from build123d import *

# Parameters (mm, degrees)
F0_W     = 10
F0_H     = 10
F0_W_2   = 8
F0_H_2   = 8
F1_DEPTH = 250
F2_R     = 1.5
F4_DEPTH = 25
F3_R     = 1.5
F3_R_2   = 2.5
F5_DEPTH = 25


with BuildPart() as f1:
    # F0 (on Front) → F1 (new body)
    with BuildSketch(Plane.XZ):
        Rectangle(F0_W, F0_H)
        Rectangle(F0_W_2, F0_H_2, mode=Mode.SUBTRACT)
    extrude(amount=F1_DEPTH)

    # F2 (on face) → F4 (cut)
    with BuildSketch(Plane.YZ.offset(5)):
        with Locations((-140.5, -1)):
            Circle(F2_R)
        with Locations((-109.5, -1)):
            Circle(F2_R)
        with Locations((-235, 0)):
            Circle(F2_R)
        with Locations((-15, 0)):
            Circle(F2_R)
    extrude(amount=-F4_DEPTH, mode=Mode.SUBTRACT)

    # F3 (on face) → F5 (cut)
    with BuildSketch(Plane.XY.offset(5)):
        with Locations((0, -245)):
            Circle(F3_R)
        with Locations((0, -5)):
            Circle(F3_R)
        with Locations((0, -215)):
            Circle(F3_R_2)
        with Locations((0, -189)):
            Circle(F3_R_2)
        with Locations((0, -61)):
            Circle(F3_R_2)
        with Locations((0, -35)):
            Circle(F3_R_2)
    extrude(amount=-F5_DEPTH, mode=Mode.SUBTRACT)


solid = f1.part
Input: part model. Units: mm. Frame: model coordinates. A direction names the side the tool comes from. Coordinates: 2 decimals unless noted, no trailing zeros. Loops run counter-clockwise (first coordinate to the right, second up) from the corner with the lowest first, then second, coordinate; pieces in that order, holes last. Notation, with made-up numbers: (-5, 12) - (37, 12) arc R5 ccw to (37, 19) - close; hole circle Ø8 at (72, 83). An arc over 180 degrees is marked (long way). Answer in a Markdown table with one row per item. Add a question column.
Item 1: Section query B-B on y = -45.5. Return the cut outline in (x, z).
Item 2: Section query A-A on y = -189. Return the cut outline in (x, z).
Item 3: Contact query for a flat-ended pin moving along its axis: P1, Ø3, axis at x = -0.5, z = -1.5, coming from the -Y side. Output: stop coordinate, or through.
Item 4: Mould query, pull axis Y, two halves, no side actions, for faces 1 (the cylindrical face through (-0.33, -186.52, 4.51)), 2 (the cylindrical face through (1.34, -32.89, 4.51)), 3 (the flat face through (0, -123, 5)), 4 (the flat face through (-4.5, -250, 0.1)). Classes: released by +Y, released by -Y, zero draft, split by the parting line, or undercut.
Item 5: Line query: line 1 along Z through (x, y) = (-2.75, -77.5); line 2 along Z through (x, y) = (-4.2, -235). Output: solid intervals per line, ascending. Write a range as [from, to].
Item 6: Access query for faces 5 (the cylindrical face through (-0.33, -186.52, -4.49)), 6 (the flat face through (4, -123, 0)). Directions: +Z, -Z, +X, -X, +Y, -Y. A direction counts if a zero-diameter tool reaches every point of the face in a straight line with its end or side. Return the directions, or none.
Recorded:
| question | item | result |
|---|---|---|
| 1 | outline | (-5, -5) - (5, -5) - (5, 5) - (-5, 5) - close; hole (-4, -4) - (4, -4) - (4, 4) - (-4, 4) - close |
| 2 | outline | (-5, -5) - (-2.5, -5) - (-2.5, -4) - (-4, -4) - (-4, 4) - (-2.5, 4) - (-2.5, 5) - (-5, 5) - close; (2.5, -5) - (5, -5) - (5, 5) - (2.5, 5) - (2.5, 4) - (4, 4) - (4, -4) - (2.5, -4) - close |
| 3 | P1 | through |
| 4 | face 1 | undercut |
| 4 | face 2 | undercut |
| 4 | face 3 | zero draft |
| 4 | face 4 | released by -Y |
| 5 | line 1 | [-5, -4], [4, 5] |
| 5 | line 2 | [-5, -1.5], [1.5, 5] |
| 6 | face 5 | +Z, -Z |
| 6 | face 6 | +Y, -Y |
